Input: part model. Units: mm. Frame: model coordinates. A direction names the side the tool comes from. Round coordinates to 2 decimals unless told otherwise and drop trailing zeros. Loops run counter-clockwise (first coordinate to the right, second up) from the corner with the lowest first, then second, coordinate; pieces in that order, holes last.
(1) Cut plane C-C, the plane z = 5. Output: boundary loops of the cut face in (x, y) (3 decimals), and give its area (3 significant figures).
(2) Draft query along X for faces 1 (the face through (3.84, 1.21, 4.86)), 2 (the face through (2, 5, 3)), 3 (the face through (5.641, -1.297, 0.986)). Return one class per face: released by +X, released by -X, zero draft, split by the parting line, or undercut.
(3) Access query for faces 4 (the face through (0, 0, 6.25)), 5 (the face through (0, 8.2, 2)). Directions: +Z, -Z, +X, -X, +Y, -Y. A direction counts if a zero-diameter tool reaches every point of the face in a straight line with its end or side. Return the directions, or none.
(4) First-contact query: pin 1 Ø3 at (y, z) = (6, 1) entering from +X; pin 2 Ø1 at (y, z) = (-2.5, 1) entering from -X; pin 3 Ø1.5 at (x, z) = (1.5, 5.5) entering from +Y; pin 4 Ø1.5 at (y, z) = (-6.5, 5) entering from +X. Flat tips, straight axial feed; report the tip coordinate or a pass-through.
(5) Line query: line 1 (Y direction, x = -3.75, z = 0.5); line 2 (Z direction, x = -5.25, y = -4.5); line 3 (Z direction, x = 7, y = -1). Output: solid intervals per line, ascending.
(6) Cut plane A-A, the plane z = 1. Give the number of separate pieces and of enclosed holes in the cut face, and give its area (3 significant figures).
from build123d import *

# Parameters (mm, degrees)
F0_R     = 11
F1_DEPTH = 3
F2_R     = 2
F3_R     = 5
F3_R_2   = 4.025
F4_DEPTH = 0.5
F5_DEPTH = 3.25
F6_R     = 3.1762732241
F6_R_2   = 2.4567004545
F6_R_3   = 1.9037122254
F6_R_4   = 1.3077812171
F7_DEPTH = 2
F8_R     = 0.7242640687


with BuildPart() as f1:
    # F0 (on Top) → F1 (new body)
    with BuildSketch(Plane.XY):
        Circle(F0_R)
    extrude(amount=F1_DEPTH)

    # F2
    f2_edges = [f1.edges().sort_by_distance(p)[0] for p in [
        (-11, 0, 0),
    ]]
    fillet(f2_edges, radius=F2_R)

    # F3 (on face) → F4 (join)
    with BuildSketch(Plane.XY.offset(3)):
        Circle(F3_R)
        Circle(F3_R_2, mode=Mode.SUBTRACT)
    extrude(amount=F4_DEPTH)

    # F5 (add): a face of the model
    f5_faces = [f1.faces().sort_by_distance(p)[0] for p in [
        (0, 0, 3),
    ]]
    extrude(f5_faces, amount=F5_DEPTH)

    # F6 (on face) → F7 (cut)
    with BuildSketch(Plane(origin=(0, 0, 0), x_dir=(1, 0, 0), z_dir=(0, 0, -1))):
        with Locations((-5.3061908111, 1.2858043192)):
            Circle(F6_R)
        with Locations((-5.3061908111, 1.2858043192)):
            Circle(F6_R_2, mode=Mode.SUBTRACT)
        with BuildLine():
            ThreePointArc((0.9619368017, -0.7183409795), (-1.1922548582, 0.140941571), (1.1029175948, 0.4742456667))
            Line((1.1029175948, 0.4742456667), (1.555835095, 0.8067932675))
            ThreePointArc((1.555835095, 0.8067932675), (-1.7466329927, 0.1442615964), (1.4023820255, -1.0511245759))
            Line((1.4023820255, -1.0511245759), (0.9619368017, -0.7183409795))
        make_face()
        Polygon((2.5934469886, 1.7158896108), (1.797987935, 1.7044660048), (1.8175899449, 1.0339289438), (2.6010603178, 1.0339289438), (2.6010603178, -1.6414519632), (3.2636339311, -1.6414519632), (3.2636339311, 1.0350090452), (3.9116484113, 1.0350090452), (3.9116484113, 1.688883407), (3.2656819094, 1.688883407), (3.2656819094, 2.9203571675), (2.5934469886, 2.5919371012), align=None)
        with Locations((5.8113215491, 0)):
            Circle(F6_R_3)
        with Locations((5.8113215491, 0)):
            Circle(F6_R_4, mode=Mode.SUBTRACT)
        with BuildLine():
            Line((5.1257074847, 6.0719344417), (5.7329160736, 6.7912362658))
            ThreePointArc((5.7329160736, 6.7912362658), (0, 8.8874752728), (-5.7329160736, 6.7912362658))
            Line((-5.7329160736, 6.7912362658), (-5.1257074847, 6.0719344417))
            ThreePointArc((-5.1257074847, 6.0719344417), (0, 7.9461478141), (5.1257074847, 6.0719344417))
        make_face()
        with BuildLine():
            ThreePointArc((5.1257074847, -6.0719344417), (0, -7.9461478141), (-5.1257074847, -6.0719344417))
            Line((-5.1257074847, -6.0719344417), (-5.7329160736, -6.7912362658))
            ThreePointArc((-5.7329160736, -6.7912362658), (0, -8.8874752728), (5.7329160736, -6.7912362658))
            Line((5.7329160736, -6.7912362658), (5.1257074847, -6.0719344417))
        make_face()
    extrude(amount=-F7_DEPTH, mode=Mode.SUBTRACT)

    # F8
    f8_edges = [f1.edges().sort_by_distance(p)[0] for p in [
        (-11, 0, 3),
    ]]
    fillet(f8_edges, radius=F8_R)


solid = f1.part
Reported:
1. outline: circle Ø8.05 at (0, 0)
1. area: 50.9 mm2
2. face 1: split by the parting line
2. face 2: zero draft
2. face 3: undercut
3. face 4: +Z, +X, -X, +Y, -Y
3. face 5: -Z
4. pin 1: stops at x = 9.94
4. pin 2: stops at x = -10.68
4. pin 3: stops at y = 3.95
4. pin 4: passes through
5. line 1: y = -9.62 to -8.06, -7.01 to -4.05, -3.19 to 0.62, 1.48 to 7.01, 8.06 to 9.62
5. line 2: z = 0 to 3
5. line 3: z = 2 to 3
6. separate pieces: 3
6. enclosed holes: 6
6. area: 313 mm2
